The model under review builds one solid part; all positions refer to its coordinate system, in mm. A direction names the side the tool comes from. Round coordinates to 2 decimals unless told otherwise and drop trailing zeros. Write each loop counter-clockwise with the first axis right and the second up, starting at its lowest first coordinate (ties: lowest second). Pieces come first, ordered by that corner, then holes. Notation, with made-up numbers: M 56,32.25 L 65,32.25 A38 cw 65,71.25 Z; hole C 73.25,-32 d7. An arc over 180 degrees is marked long. One line per item, written item: value. Start each with the question number.
1) Take a section at D-D, the plane y = -85. Write out the cut boundary in (x, z) (3 decimals).
2) Take a section at A-A, the plane z = 16. Write out the cut boundary in (x, y).
3) Tool access review of faces 4 (the face through (49.523, -87, 25)), 5 (the face through (32.17, -65.07, 25.76)), 6 (the face through (-43.103, -86.912, 3.176)), 7 (the face through (-39, -77.898, 25)): name each direction out of +Z, -Z, +X, -X, +Y, -Y from which nothing blocks a thin tool from reaching the whole face with its end or side.
4) Take a section at C-C, the plane y = 36. Write out the cut boundary in (x, z).
5) Mouldability with a two-part tool opening along X and no side actions: class faces 1 (the face through (-44, -58.108, 26)), 2 (the face through (-32.17, -65.07, 25.76)), 3 (the face through (43.103, -86.912, 47.624)) as +X half, -X half, draft (parallel to the pull), parting line (faces both ways), or undercut.
6) For P1, Ø4, axis at y = 8.5, z = 18, coming from the -X side; P2, Ø4, axis at y = -12.5, z = 36.5, coming from the -X side; P3, Ø5, axis at x = 18.5, z = 7, coming from the +Y side, all flat-tipped, find the tip position at first contact; note any pin that passes through.
7) Take a section at B-B, the plane x = 0. Write out the cut boundary in (y, z), and give its area (3 significant figures).
8) Wall thickness on probe 1 along X at (y, z) = (-82.5, 12); probe 2 along X at (y, z) = (0, 29); probe 3 along Y at (x, z) = (38, 3): over which ranges is each line inside the solid? List them lowest first.
from build123d import *

# Parameters (mm, degrees)
BOSS_EXTRUDE1_DEPTH     = 50.8
CUT_EXTRUDE1_DEPTH      = 25.4
CUT_EXTRUDE2_DEPTH      = 72.136
CUT_EXTRUDE3_DEPTH      = 113.284
CUT_EXTRUDE3_DEPTH_BACK = 90.424
SKETCH5_R               = 1.27


with BuildPart() as part:
    # Sketch2 → Boss-Extrude1 (new body)
    with BuildSketch(Plane.XY):
        with BuildLine():
            Line((31.743188487, -77.898004197), (49.523188487, -77.898004197))
            Line((49.523188487, -77.898004197), (49.523188487, -95.678004197))
            Line((49.523188487, -95.678004197), (-49.523188487, -95.678004197))
            Line((-49.523188487, -95.678004197), (-49.523188487, -77.898004197))
            Line((-49.523188487, -77.898004197), (-31.743188487, -77.898004197))
            ThreePointArc((-31.743188487, -77.898004197), (-27.358253154, -76.140916358), (-25.4, -71.842048969))
            ThreePointArc((-25.4, -71.842048969), (-73.310915254, -20.783399738), (-59.324614565, 47.822903578))
            ThreePointArc((-59.324614565, 47.822903578), (0, 76.2), (59.324614565, 47.822903578))
            ThreePointArc((59.324614565, 47.822903578), (73.310915254, -20.783399738), (25.4, -71.842048969))
            ThreePointArc((25.4, -71.842048969), (27.358253154, -76.140916358), (31.743188487, -77.898004197))
        make_face()
        with BuildLine():
            ThreePointArc((-35.199271309, 28.37492279), (0, -45.212), (35.199271309, 28.37492279))
            ThreePointArc((35.199271309, 28.37492279), (0, 45.212), (-35.199271309, 28.37492279))
        make_face(mode=Mode.SUBTRACT)
    extrude(amount=BOSS_EXTRUDE1_DEPTH)

    # Sketch3 → Cut-Extrude1 (cut)
    with BuildSketch(Plane.XZ.offset(95.678004197)):
        with BuildLine():
            Line((-39.998188487, 44.45), (-39.998188487, 6.35))
            ThreePointArc((-39.998188487, 6.35), (-43.173188487, 3.175), (-46.348188487, 6.35))
            Line((-46.348188487, 6.35), (-46.348188487, 44.45))
            ThreePointArc((-46.348188487, 44.45), (-43.173188487, 47.625), (-39.998188487, 44.45))
        make_face()
        with BuildLine():
            Line((46.348188487, 44.45), (46.348188487, 6.35))
            ThreePointArc((46.348188487, 6.35), (43.173188487, 3.175), (39.998188487, 6.35))
            Line((39.998188487, 6.35), (39.998188487, 44.45))
            ThreePointArc((39.998188487, 44.45), (43.173188487, 47.625), (46.348188487, 44.45))
        make_face()
    extrude(amount=-CUT_EXTRUDE1_DEPTH, mode=Mode.SUBTRACT)

    # Sketch4 → Cut-Extrude2 (cut)
    with BuildSketch(Plane.XY.offset(50.8)):
        with BuildLine():
            Line((25.4, -71.842048969), (39.134215056, -58.107833913))
            Line((39.134215056, -58.107833913), (49.294215056, -58.107833913))
            ThreePointArc((49.294215056, -58.107833913), (40.1915566, -69.92359541), (25.4, -71.842048969))
        make_face()
        with BuildLine():
            Line((-25.400000099, -71.842048964), (-39.134215677, -58.107833386))
            Line((-39.134215677, -58.107833386), (-49.294215677, -58.107833386))
            ThreePointArc((-49.294215677, -58.107833386), (-40.191557069, -69.923595252), (-25.400000099, -71.842048964))
        make_face()
    extrude(amount=-CUT_EXTRUDE2_DEPTH, mode=Mode.SUBTRACT)

    # Sketch5 → Cut-Extrude3 (cut, two sides: drawn at the far end of the back side and taken through both)
    with BuildSketch(Plane(origin=(0, 0, 0), x_dir=(0, 0, -1), z_dir=(1, 0, 0)).offset(-CUT_EXTRUDE3_DEPTH_BACK)):
        with Locations(Location((-25.4, 0, 0), (0, 0, 180))):
            Circle(SKETCH5_R)
    extrude(amount=CUT_EXTRUDE3_DEPTH + CUT_EXTRUDE3_DEPTH_BACK, mode=Mode.SUBTRACT)


solid = part.part
Checked values:
1. outline: M -49.523,0 L 49.523,0 L 49.523,50.8 L -49.523,50.8 Z; hole M -46.348,6.35 A3.175 ccw -39.998,6.35 L -39.998,44.45 A3.175 ccw -46.348,44.45 Z; hole M 39.998,6.35 A3.175 ccw 46.348,6.35 L 46.348,44.45 A3.175 ccw 39.998,44.45 Z
2. outline: M -49.52,-95.68 L -46.35,-95.68 L -46.35,-77.9 L -49.52,-77.9 Z; M -49.29,-58.11 L -39.13,-58.11 L -25.4,-71.84 A6.35 cw -31.74,-77.9 L -40,-77.9 L -40,-95.68 L 40,-95.68 L 40,-77.9 L 31.74,-77.9 A6.35 cw 25.4,-71.84 L 39.13,-58.11 L 49.29,-58.11 A76.2 ccw long Z; M 46.35,-95.68 L 49.52,-95.68 L 49.52,-77.9 L 46.35,-77.9 Z; hole C 0,0 d90.42
3. face 4: +Z, -Z, +X, -Y
3. face 5: +Z, -Z, +X
3. face 6: -Y
3. face 7: +Z, -Z, -X
4. outline: M -67.16,0 L -27.35,0 L -27.35,50.8 L -67.16,50.8 Z; M 27.35,0 L 67.16,0 L 67.16,50.8 L 27.35,50.8 Z
5. face 1: draft
5. face 2: -X half
5. face 3: undercut
6. P1: stops at x = -75.92
6. P2: stops at x = -75.47
6. P3: stops at y = 74.5
7. outline: M -95.68,0 L -45.21,0 L -45.21,50.8 L -95.68,50.8 Z; M 45.21,0 L 76.2,0 L 76.2,50.8 L 45.21,50.8 Z
7. area: 4,140 mm2
8. probe 1: x = -49.52 to -46.35, -40 to 40, 46.35 to 49.52
8. probe 2: x = -76.2 to -45.21, 45.21 to 76.2
8. probe 3: y = -95.68 to -77.9, -59.24 to -24.5, 24.5 to 66.05
